Check sheet for the modelled part. Datum: model origin and axes. Units: mm. Give positions to 0.01 mm unless a question says otherwise; leave off trailing zeros. Write each loop counter-clockwise with the first axis right and the second up, starting at its lowest first coordinate (ties: lowest second). Pieces come first, ordered by that corner, then holes.
from build123d import *

# Parameters (mm, degrees)
F1_DEPTH = 3.175


# Not quite as in the source:
# - a feature names something its author has since deleted; it is built from what else it names


with BuildPart() as f1:
    # F0 (on Front) → F1 (new body)
    with BuildSketch(Plane.XZ):
        Polygon((-57.15, -43.18), (57.15, -43.18), (57.15, -19.05), (60.325, -19.05), (60.325, 19.05), (57.15, 19.05), (57.15, 43.18), (19.05, 43.18), (19.05, 40.005), (-19.05, 40.005), (-19.05, 43.18), (-57.15, 43.18), (-57.15, 19.05), (-60.325, 19.05), (-60.325, 0), (-60.325, -19.05), (-57.15, -19.05), align=None)
    extrude(amount=F1_DEPTH)


solid = f1.part
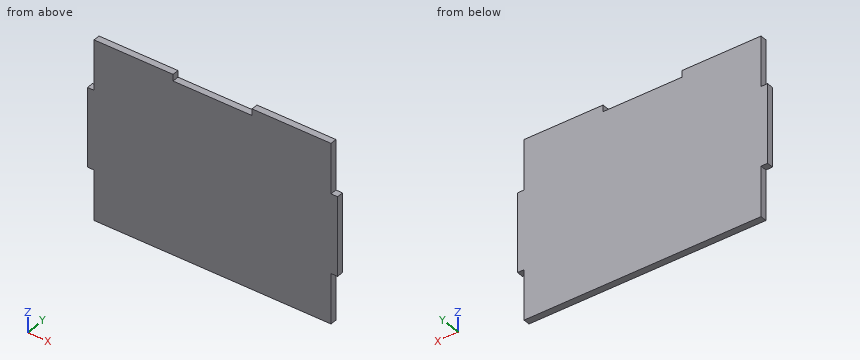
1) Sectioned sample at C-C on x = -6. Record the boundary of the cut face in (y, z) (3 decimals).
2) Sectioned sample at B-B on z = -36. Record the boundary of the cut face in (x, y) (3 decimals), then the cut area to 3 significant figures.
3) Gauge pin test, flat ends, axial feed: pin 1 (1.6 mm diameter, centred on y = -1.5, z = 41, fed in from -X); pin 2 (1.6 mm diameter, centred on x = -58, y = -2, fed in from -Z); pin 3 (1 mm diameter, centred on x = -6, y = -2, fed in from +Z) (3 decimals). Record the tip position at first contact, or that the pin passes through.
4) Scan lines: L1, parallel to X at y = -2.95, z = -20; L2, parallel to Z at x = -10.5, y = -1.35 (3 decimals). Record each from-to range of solid material in increasing order.
5) Sectioned sample at A-A on y = -1.6. Record the boundary of the cut face in (x, z) (3 decimals).
Answers below:
1. outline: (-3.175, -43.18) - (0, -43.18) - (0, 40.005) - (-3.175, 40.005) - close
2. outline: (-57.15, -3.175) - (57.15, -3.175) - (57.15, 0) - (-57.15, 0) - close
2. area: 363 mm2
3. pin 1: stops at x = -57.15
3. pin 2: stops at z = -19.05
3. pin 3: stops at z = 40.005
4. L1: x = -57.15 to 57.15
4. L2: z = -43.18 to 40.005
5. outline: (-60.325, -19.05) - (-57.15, -19.05) - (-57.15, -43.18) - (57.15, -43.18) - (57.15, -19.05) - (60.325, -19.05) - (60.325, 19.05) - (57.15, 19.05) - (57.15, 43.18) - (19.05, 43.18) - (19.05, 40.005) - (-19.05, 40.005) - (-19.05, 43.18) - (-57.15, 43.18) - (-57.15, 19.05) - (-60.325, 19.05) - close
